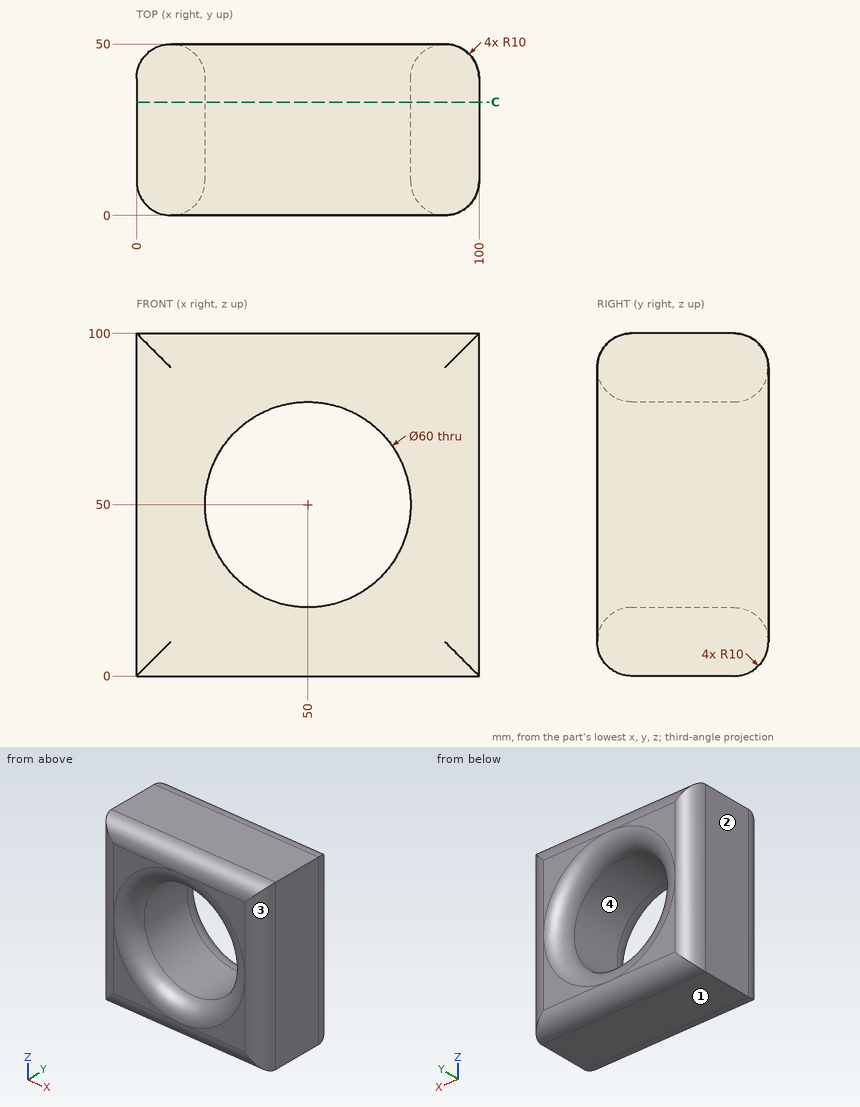
Check sheet for the drawn part. Datum: minimum x, y, z corner. Units: mm. Give positions to 0.01 mm unless a question says otherwise; leave off trailing zeros. Order: outer loops, then holes, each group sorted by start corner. A loop starts at its lowest first (then second) coordinate and runs counter-clockwise, first axis right, second up. Notation, with made-up numbers: (-32.5, 89.25) -> (-0.5, 89.25) arc R19 cw to (-0.5, 104.25) -> close; hole circle Ø2 at (26.25, 20). An arc over 180 degrees is marked (long way). Use a Markdown table: item, result.
1) Material ranges on probe 1 along Z at (x, y) = (50, 26); probe 2 along Z at (x, y) = (74, 18.5); probe 3 along X at (y, z) = (30, 75.5), recorded low to high.
Results:
| item | result |
|---|---|
| probe 1 | 0 to 20, 80 to 100 |
| probe 2 | 0 to 32, 68 to 100 |
| probe 3 | 0 to 34.2, 65.8 to 100 |
2) Section check C-C, the plane y = 33. Record the boundary of the cut face in (x, z), then the cut area to 3 significant figures.
Results:
| item | result |
|---|---|
| outline | (0, 0) -> (100, 0) -> (100, 100) -> (0, 100) -> close; hole circle Ø60 at (50, 50) |
| area | 7,170 mm² |
3) Depth check by flat-ended pin: pin 1 Ø1 at (x, z) = (73.5, 74.5) entering from -Y; pin 2 Ø5 at (x, y) = (25, 42) entering from -Z; pin 3 Ø12 at (x, z) = (26.5, 28.5) entering from +Y. Enter the tip coordinate at first touch or a pass-through.
Results:
| item | result |
|---|---|
| pin 1 | y = 1.68 |
| pin 2 | z = 0 |
| pin 3 | y = 49.77 |
4) Mould release check, pull along X, two halves, no side actions. Record for the marked faces 1, 2, 3 and 4: pulls with the +X half, pulls with the -X half, needs draft (parallel to the pull), parting line crosses it, or undercut.
Results:
| item | result |
|---|---|
| face 1 | needs draft |
| face 2 | pulls with the -X half |
| face 3 | pulls with the +X half |
| face 4 | undercut |
